Autodesk Inventor part; units mm, degrees
ref_plane "YZ Plane" through (0, 0, 0) normal (1, 0, 0) x (0, 1, 0)
ref_plane "XZ Plane" through (0, 0, 0) normal (0, 1, 0) x (-1, 0, 0)
ref_plane "XY Plane" through (0, 0, 0) normal (0, 0, 1) x (1, 0, 0)
sketch "Sketch1" plane through (0, 0, 0) normal (0, 1, 0) x (-1, 0, 0)
  circle A0 centre (0, 0) radius 4.75
  dimension "d0" = 9.5
extrude "Extrusion1" add sketch "Sketch1" along normal blind 1.5
chamfer "Chamfer1" distance 0.8 distance2 1.2 1 edges at (4.75, 1.5, 0) measured on face at (-1.1851, 1.5, -1.0499)
sketch "Sketch2" plane through (0, 0, 0) normal (0, -1, 0) x (1, 0, 0)
  circle A0 centre (0, 0) radius 4
  dimension "d6" = 8
extrude "Extrusion2" add sketch "Sketch2" along normal blind 12
chamfer "Chamfer2" distance 0.8 angle 45 1 edges at (-4, -12, 0)
thread "Thread1"
sketch "Sketch3" plane through (0, -12, 0) normal (0, -1, 0) x (1, 0, 0)
  circle A0 centre (0, 0) radius 3.2
extrude "Extrusion3" add sketch "Sketch3" along normal blind 5
sketch "Sketch4" plane through (0, -17, 0) normal (0, -1, 0) x (1, 0, 0)
  line L0 (1.75, -1.75) -> (-1.75, -1.75)
  line L1 (1.75, -1.75) -> (-1.75, 1.75) construction
  line L2 (-1.75, -1.75) -> (1.75, 1.75) construction
  line L3 (0, 6.1884) -> (0, -7.5413) construction
  line L4 (-9.3951, 0) -> (6.4878, 0) construction
  line L5 (1, 1.5) -> (-1, 1.5)
  line L6 (-1, 1.5) -> (-1, 2)
  line L7 (-1, 2) -> (1, 2)
  line L8 (1, 2) -> (1, 1.5)
  line L9 (1, 1.5) -> (-1, 2) construction
  line L10 (-1, 1.5) -> (1, 2) construction
  line L11 (2, -1) -> (1.5, -1)
  line L12 (1.5, -1) -> (1.5, 1)
  line L13 (1.5, 1) -> (2, 1)
  line L14 (2, 1) -> (2, -1)
  line L15 (2, -1) -> (1.5, 1) construction
  line L16 (1.5, -1) -> (2, 1) construction
  line L17 (-1.5, -1) -> (-2, -1)
  line L18 (-2, -1) -> (-2, 1)
  line L19 (-2, 1) -> (-1.5, 1)
  line L20 (-1.5, 1) -> (-1.5, -1)
  line L21 (-1.5, -1) -> (-2, 1) construction
  line L22 (-2, -1) -> (-1.5, 1) construction
  line L23 (1.75, 1.75) -> (1.75, 1)
  line L24 (1.75, -1) -> (1.75, -1.75)
  line L25 (-1.75, -1.75) -> (-1.75, -1)
  line L26 (-1.75, 1) -> (-1.75, 1.75)
  line L27 (-1.75, 1.75) -> (-1, 1.75)
  line L28 (1, 1.75) -> (1.75, 1.75)
  point P0 (0, 0)
  point P1 (0, 0)
  point P2 (0, 0)
  dimension "d16" = 3.5
  dimension "d17" = 3.5
  dimension "d18" = 2
  dimension "d19" = 0.5
  dimension "d20" = 0.5
  dimension "d21" = 2
  dimension "d22" = 0.5
  dimension "d23" = 2
extrude "Extrusion4" add sketch "Sketch4" along normal blind 6 contours L11 L12 L13 L14 | L17 L18 L19 L20 | L8 L5 L6 L7
fillet "Fillet1" radius 1 6 edges at (-1.75, -23, 1) (-1.75, -23, -1) (-1, -23, 1.75) (1, -23, 1.75) (1.75, -23, 1) (1.75, -23, -1)
properties part number "LED Indicator Farnell 19100054"
Can you work these out from the model? Positions are in its coordinate system, mm. A direction names the side the tool comes from. Coordinates: 2 decimals unless noted, no trailing zeros. Loops run counter-clockwise (first coordinate to the right, second up) from the corner with the lowest first, then second, coordinate; pieces in that order, holes last. Notation, with made-up numbers: M 69.25,-8 L 92.25,-8 A28 cw 92.25,24 Z; hole C 26,75 d8. An arc over 180 degrees is marked long. Return JSON: item names as keys, results as strings. Group by question number.
Item 1: On a 3-axis mill with a long thin cutter (end or side, diameter ignored), from which of +Z, -Z, +X, -X, +Y, -Y can I reach the whole of each face in a straight line? I mean faces 5 (the cylindrical face through (-0.867, -5.522, 3.905)), 6 (the flat face through (0, -20, 1.5)), 7 (the flat face through (-2, -20, 0)). Say none if no direction works.
Item 2: Imagine slicing it at B-B (y = -13.25). Please give me the cut outline in (x, z), and give its area (3 significant figures).
Item 3: I'm going to push flat-ended pins straight in: pin 1 Ø3 at (x, y) = (-3.5, -4.5) entering from -Z; pin 2 Ø3 at (x, y) = (-1.5, -11) entering from -Z; pin 3 Ø1 at (y, z) = (-20.5, -0.5) entering from +X; pin 4 Ø5 at (x, z) = (1.5, -0.5) entering from -Y. Where does each tip first touch, or does it pass through?
Item 4: If I drill on L1, parallel to Y at x = 0.75, z = -1.5; L2, parallel to Z at x = 0.5, y = -21.25; L3, parallel to X at y = -4.5, z = -2.25, over which ranges is the centre line in solid material (lowest first)? Write a range as from..to.
Item 5: Thinking about a two-plate mould opening in X: for faces 1 (the flat face through (1.5, -20, 0)), 2 (the cylindrical face through (-2.539, -14.465, 1.947)), 3 (the flat face through (4, 0, -2)), 4 (the flat face through (0, -17, 0)), which applies, released by +X, released by -X, zero draft, split by the parting line, or undercut?
Item 6: Imagine slicing it at A-A (y = -20.5). Please give me the cut outline in (x, z), and give its area (3 significant figures).
Verdict:
{
 "1": {"face 5": "-Y", "face 6": "-Z, +X, -X, -Y", "face 7": "+Z, -Z, -X, -Y"},
 "2": {"outline": "C 0,0 d6.4", "area": "32.2 mm^2"},
 "3": {"pin 1": "stops at z = -3.46", "pin 2": "stops at z = -4", "pin 3": "stops at x = 2", "pin 4": "stops at y = -23"},
 "4": {"L1": "y = -17..1.5", "L2": "z = 1.5..2", "L3": "x = -3.31..3.31"},
 "5": {"face 1": "undercut", "face 2": "split by the parting line", "face 3": "zero draft", "face 4": "undercut"},
 "6": {"outline": "M -2,-1 L -1.5,-1 L -1.5,1 L -2,1 Z; M -1,1.5 L 1,1.5 L 1,2 L -1,2 Z; M 1.5,-1 L 2,-1 L 2,1 L 1.5,1 Z", "area": "3.00 mm^2"}
}
